The listing builds one solid part. Answer for the finished solid, in the listing's coordinates (mm). Face numbers are marked on the shaded views. A direction names the side the tool comes from. Coordinates: 2 decimals unless noted, no trailing zeros. Return JSON: item names as keys, results as strings. Group by question number.
1. Each of these flat-tipped pins is pushed along its axis until it touches: P1, Ø5, axis at y = -74.43, z = -54.08, coming from the +X side; P2, Ø12, axis at x = 234, y = -10.5, coming from the +Z side; P3, Ø3, axis at y = 74.43, z = 54.08, coming from the -X side; P4, Ø6, axis at x = 169.5, y = -47, coming from the -Z side. Where does it stop, or does it pass through?
2. Which of the six approach directions +Z, -Z, +X, -X, +Y, -Y give full straight-line access (tool end or side, diameter ignored) to the marked faces 1 and 2?
3. Find the intervals of material crossed by line 1 along Z through (x, y) = (3.15, 0); line 2 along Z through (x, y) = (2, 0); line 3 along X through (y, z) = (85, 49), in increasing order.
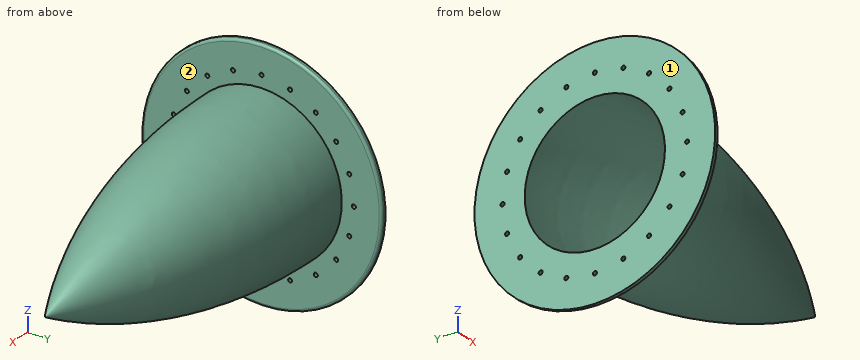
Autodesk Fusion 360 part; units mm, degrees
sketch "Sketch1" plane through (0, 0, 0) normal (0, 1, 0) x (1, 0, 0)
  line L0 (284.8084, 0) -> (305, 0) construction
  line L1 (305, 0) -> (305, -120) construction
  line L2 (305, -120) -> (0, -120) construction
  line L3 (0, -120) -> (0, -69.9357) construction
  line L4 (0, -69.9357) -> (0, -120)
  line L5 (5, -120) -> (5, -80.02)
  line L6 (0, -120) -> (5, -120)
  arc A0 (5, -80.02) -> (305, 0) centre (11.9649, 496.2375) ccw
  arc A1 (0, -69.9357) -> (284.8084, 0) centre (11.9649, 496.2375) ccw
  line L7 (305, 0) -> (303.3901, 0)
  line L8 (305, 0) -> (300.6101, 0)
  line L9 (305, 0) -> (284.8084, 0)
  dimension "d1" = 120
  dimension "d3" = 5
  dimension "d5" = 80.02
  dimension "d6" = 305
revolve "Revolve1" add sketch "Sketch1" angle 360 about axis through (1.75, 0, 0) along (1, 0, 0)
fillet "Fillet1" radius 2.5 1 edges at (5, -43.3939, -111.8793)
sketch "Sketch2" plane through (0, 0, 0) normal (-1, 0, 0) x (0, -1, 0)
  circle A0 centre (0, 0) radius 120
  circle A1 centre (0, 0) radius 69.9357
  line L0 (0, 0) -> (0, 143.5123) construction
  circle A2 centre (0, 92) radius 2
  dimension "d11" = 4
  dimension "d12" = 92
extrude "Extrude1" cut sketch "Sketch2" along normal mid plane 12 contours A2
pattern_circular "C-Pattern1" count 20 over 360 about axis through (1.75, 0, 0) along (1, 0, 0) of "Extrude1"
The answers:
{
 "1": {"P1": "stops at x = 5", "P2": "stops at z = 36.96", "P3": "passes through", "P4": "stops at z = -38.2"},
 "2": {"face 1": "+Z, -Z, -X, +Y, -Y", "face 2": "+X"},
 "3": {"line 1": "z = -119.91 to -94, -90 to -69.99, 69.99 to 90, 94 to 119.91", "line 2": "z = -120 to -94, -90 to -69.97, 69.97 to 90, 94 to 120", "line 3": "x = 0 to 5"}
}
